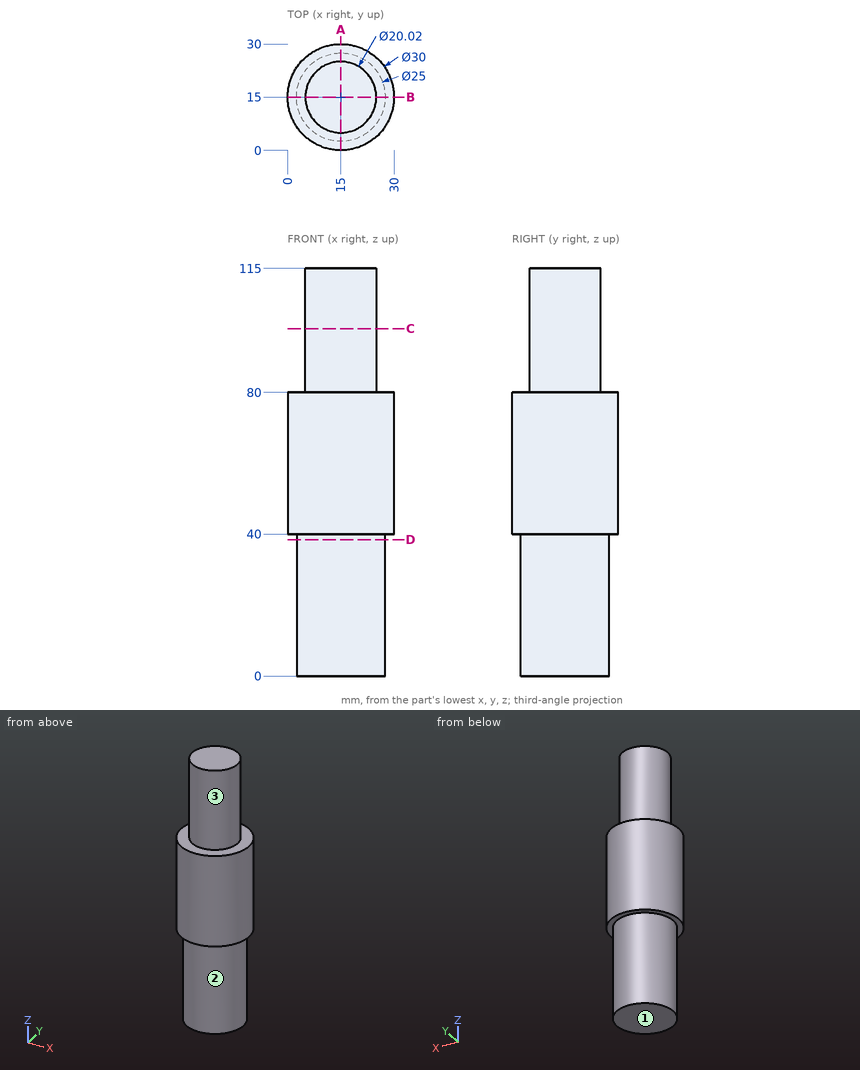
Source: three-view drawing plus pictorial views. Frame: mm from the lowest corner of the part. A direction names the side the tool comes from. Round coordinates to 2 decimals unless told otherwise and drop trailing zeros. Order: outer loops, then holes, each group sorted by start corner. A loop starts at its lowest first (then second) coordinate and runs counter-clockwise, first axis right, second up. Notation, with made-up numbers: (-36.5, -29.5) - (-30.5, -29.5) arc R19 cw to (-30.5, -23.5) - close; hole circle Ø10 at (86, -20). An arc over 180 degrees is marked (long way). Write each question's results on one line, items separated by ' | '.
Item 1: First-contact query: pin 1 Ø3 at (y, z) = (6, 98.5) entering from -X; pin 2 Ø3 at (x, z) = (4, 57) entering from -Y; pin 3 Ø2 at (x, z) = (8.5, 74) entering from -Y. Flat tips, straight axial feed; report the tip coordinate or a pass-through.
Completed:
pin 1: x = 8.37 | pin 2: y = 3.39 | pin 3: y = 1.04
Item 2: Section A-A, the plane x = 15. Return the cut outline in (y, z), and give its area (3 significant figures).
Completed:
outline: (0, 40) - (2.5, 40) - (2.5, 0) - (27.5, 0) - (27.5, 40) - (30, 40) - (30, 80) - (25.01, 80) - (25.01, 115) - (4.99, 115) - (4.99, 80) - (0, 80) - close | area: 2,900 mm^2
Item 3: Material intervals for line 1 along Z through (x, y) = (25, 9); line 2 along Z through (x, y) = (18.25, 28); line 3 along X through (y, z) = (12, 109), sorted ascending. Write a range as [from, to].
Completed:
line 1: [0, 80] | line 2: [40, 80] | line 3: [5.45, 24.55]
Item 4: Section C-C, the plane z = 98. Return the cut outline in (x, y), and give its area (3 significant figures).
Completed:
outline: circle Ø20.02 at (15, 15) | area: 315 mm^2
Item 5: Reachability of the marked faces 1, 2 and 3 from +Z, -Z, +X, -X, +Y, -Y: full face, straight path, thin tool, end or side. Return the list, or none.
Completed:
face 1: -Z, +X, -X, +Y, -Y | face 2: -Z | face 3: +Z
Item 6: Section D-D, the plane z = 38.5. Return the cut outline in (x, y).
Completed:
outline: circle Ø25 at (15, 15)
